```python
from build123d import *

# Parameters (mm, degrees)
F1_DEPTH = 2.5


with BuildPart() as f1:
    # F0 (on Top) → F1 (new body, symmetric)
    with BuildSketch(Plane.XY):
        Polygon((0, 30), (-25.980762, 15), (-25.980762, -15), (0, -30), (25.980762, -15), (25.980762, 15), align=None)
        Polygon((-12.990381, -7.5), (-12.990381, 7.5), (0, 15), (12.990381, 7.5), (12.990381, -7.5), (0, -15), align=None, mode=Mode.SUBTRACT)
    extrude(amount=F1_DEPTH, both=True)


solid = f1.part
```
Can you work these out from the model? Positions are in its coordinate system, mm. A direction names the side the tool comes from. Coordinates: 2 decimals unless noted, no trailing zeros. Loops run counter-clockwise (first coordinate to the right, second up) from the corner with the lowest first, then second, coordinate; pieces in that order, holes last. Notation, with made-up numbers: (64, -22) - (107, -22) arc R19 cw to (107, 0) - close; hole circle Ø8 at (68, 58.5). An arc over 180 degrees is marked (long way). Answer as CSV lines item,"result". Start each with the question number.
1) Suppose I cut it at C-C (x = 1.5). Please give me the cut outline in (y, z), plus the area to 3 significant figures.
2) Which directions (+Z, -Z, +X, -X, +Y, -Y) give clear straight access to the entire face, cutting with the end or side of a thin tool? Please do faces 1 (the flat face through (-6.404, -11.302, 0.035)), 2 (the flat face through (13.172, 22.395, 0.035)).
3) Suppose I cut it at B-B (z = -1.8). Please give me the cut outline in (x, y).
4) Suppose I cut it at D-D (y = 25.5). Please give me the cut outline in (x, z), plus the area to 3 significant figures.
5) I need wall thicknesses on line 1 (X direction, y = 5, z = 0.8); line 2 (X direction, y = 11, z = -0.9); line 3 (Y direction, x = 4, z = -0.05). Which ranges of each line are inside material? Lowest first, please. Write a range as from..to.
6) For pin 1 (2 mm diameter, centred on x = -9, z = -1.5, fed in from -Y), with a flat end and sliding along its axis, tell me the tip position at first contact or that it passes through.
7) Suppose I cut it at A-A (y = -3). Please give me the cut outline in (x, z), plus the area to 3 significant figures.
Check result:
1,outline,"(-29.13, -2.5) - (-14.13, -2.5) - (-14.13, 2.5) - (-29.13, 2.5) - close; (14.13, -2.5) - (29.13, -2.5) - (29.13, 2.5) - (14.13, 2.5) - close"
1,area,"150 mm²"
2,face 1,"+Z, -Z"
2,face 2,"+Z, -Z, +X, +Y"
3,outline,"(-25.98, -15) - (0, -30) - (25.98, -15) - (25.98, 15) - (0, 30) - (-25.98, 15) - close; hole (-12.99, -7.5) - (0, -15) - (12.99, -7.5) - (12.99, 7.5) - (0, 15) - (-12.99, 7.5) - close"
4,outline,"(-7.79, -2.5) - (7.79, -2.5) - (7.79, 2.5) - (-7.79, 2.5) - close"
4,area,"77.9 mm²"
5,line 1,"x = -25.98..-12.99, 12.99..25.98"
5,line 2,"x = -25.98..-6.93, 6.93..25.98"
5,line 3,"y = -27.69..-12.69, 12.69..27.69"
6,pin 1,"stops at y = -25.38"
7,outline,"(-25.98, -2.5) - (-12.99, -2.5) - (-12.99, 2.5) - (-25.98, 2.5) - close; (12.99, -2.5) - (25.98, -2.5) - (25.98, 2.5) - (12.99, 2.5) - close"
7,area,"130 mm²"
